```python
from build123d import *

# Parameters (mm, degrees)
SKETCH1_R           = 3.175
BOSS_EXTRUDE1_DEPTH = 3.175


with BuildPart() as part:
    # Sketch1 → Boss-Extrude1 (new body)
    with BuildSketch(Plane.XY):
        Polygon((6.35, 12.7), (-6.35, 12.7), (-109.769758062, -271.44345), (-84.369758062, -271.44345), (-63.785953331, -214.889911296), (63.785953331, -214.889911296), (84.369758062, -271.44345), (109.769758062, -271.44345), align=None)
        Circle(SKETCH1_R, mode=Mode.SUBTRACT)
        with Locations((0, -48.55845)):
            Circle(SKETCH1_R, mode=Mode.SUBTRACT)
        with Locations((0, -202.189911296)):
            Circle(SKETCH1_R, mode=Mode.SUBTRACT)
        Polygon((54.541109381, -189.489911296), (10.527609118, -68.563813172), (-10.527609118, -68.563813172), (-54.541109381, -189.489911296), align=None, mode=Mode.SUBTRACT)
    extrude(amount=BOSS_EXTRUDE1_DEPTH)


solid = part.part
```
Input: part model. Units: mm. Frame: model coordinates. A direction names the side the tool comes from. Give positions to 0.01 mm unless a question says otherwise; leave off trailing zeros. Order: outer loops, then holes, each group sorted by start corner. A loop starts at its lowest first (then second) coordinate and runs counter-clockwise, first axis right, second up. Notation, with made-up numbers: M 35,22 L 93,22 A21 cw 93,26 Z; hole C 22,22 d4. An arc over 180 degrees is marked long. Return JSON: item names as keys, results as strings.
1) Section query D-D on z = 2.4. Output: boundary loops of the cut face in (x, y) (3 decimals).
Taken from the geometry:
{"outline": "M -109.77,-271.443 L -84.37,-271.443 L -63.786,-214.89 L 63.786,-214.89 L 84.37,-271.443 L 109.77,-271.443 L 6.35,12.7 L -6.35,12.7 Z; hole M -54.541,-189.49 L 54.541,-189.49 L 10.528,-68.564 L -10.528,-68.564 Z; hole C 0,-202.19 d6.35; hole C 0,-48.558 d6.35; hole C 0,0 d6.35"}
2) Section query A-A on x = 0. Output: boundary loops of the cut face in (y, z) (3 decimals).
Taken from the geometry:
{"outline": "M -214.89,0 L -205.365,0 L -205.365,3.175 L -214.89,3.175 Z; M -199.015,0 L -189.49,0 L -189.49,3.175 L -199.015,3.175 Z; M -68.564,0 L -51.733,0 L -51.733,3.175 L -68.564,3.175 Z; M -45.383,0 L -3.175,0 L -3.175,3.175 L -45.383,3.175 Z; M 3.175,0 L 12.7,0 L 12.7,3.175 L 3.175,3.175 Z"}
3) Access query for faces 5 (the face through (-57.336, -127.383, 1.565)), 6 (the face through (-32.226, -128.18, 1.565)), 7 (the face through (73.934, -242.771, 1.565)). Directions: +Z, -Z, +X, -X, +Y, -Y. A direction counts if a zero-diameter tool reaches every point of the face in a straight line with its end or side. Return the directions, or none.
Taken from the geometry:
{"face 5": "+Z, -Z, -X, +Y", "face 6": "+Z, -Z", "face 7": "+Z, -Z, -Y"}
4) Line query: L1, parallel to Y at x = 0, z = 1 (3 decimals); L2, parallel to X at y = -44, z = 1.7; L3, parallel to X at y = -129.5, z = 2.9. Output: solid intervals per line, ascending. Write a range as [from, to].
Taken from the geometry:
{"L1": "y = [-214.89, -205.365], [-199.015, -189.49], [-68.564, -51.733], [-45.383, -3.175], [3.175, 12.7]", "L2": "x = [-26.99, 26.99]", "L3": "x = [-58.11, -32.71], [32.71, 58.11]"}
5) Section query C-C on x = -47. Output: boundary loops of the cut face in (y, z) (3 decimals).
Taken from the geometry:
{"outline": "M -214.89,0 L -189.49,0 L -189.49,3.175 L -214.89,3.175 Z; M -168.771,0 L -98.985,0 L -98.985,3.175 L -168.771,3.175 Z"}
6) Section query B-B on y = -171.5. Output: boundary loops of the cut face in (x, z) (3 decimals).
Taken from the geometry:
{"outline": "M -73.393,0 L -47.993,0 L -47.993,3.175 L -73.393,3.175 Z; M 47.993,0 L 73.393,0 L 73.393,3.175 L 47.993,3.175 Z"}
7) Mould query, pull axis Y, two halves, no side actions, for faces 1 (the face through (58.8, -131.4, 1.6)), 2 (the face through (-41, -150, 0)), 3 (the face through (-0.69, -3.1, 1.57)), 4 (the face through (-0.688, -51.658, 1.565)). Classes: released by +Y, released by -Y, zero draft, split by the parting line, or undercut.
Taken from the geometry:
{"face 1": "released by +Y", "face 2": "zero draft", "face 3": "undercut", "face 4": "undercut"}
8) Contact query for a flat-ended pin moving along its axis: pin 1 (1.5 mm diameter, centred on x = -44.5, z = 0.5, fed in from -Y). Output: stop coordinate, or through.
Taken from the geometry:
{"pin 1": "stops at y = -214.89"}
